Source: CAD feature listing. Evaluate the final solid. Frame: model axes, mm. Face numbers are marked on the shaded views. Coordinates: 2 decimals unless noted, no trailing zeros. Order: outer loops, then holes, each group sorted by start corner. A loop starts at its lowest first (then second) coordinate and runs counter-clockwise, first axis right, second up. Notation, with made-up numbers: (-1.5, 85.5) -> (5.5, 85.5) arc R30 cw to (5.5, 112.5) -> close; hole circle Ø8 at (25, -36). An arc over 180 degrees is marked (long way). Put each result on its own line as item: value.
from build123d import *

# Parameters (mm, degrees)
SKETCH1_R               = 12.5
SKETCH1_R_2             = 9.5
BOSS_EXTRUDE1_DEPTH     = 2
SKETCH1_3_R             = 9.5
SKETCH1_3_R_2           = 5
BOSS_EXTRUDE2_DEPTH     = 41.5
CUT_EXTRUDE1_REACH      = 47.108
CUT_EXTRUDE1_END_RADIUS = 9.5
SKETCH2_R               = 2.5


with BuildPart() as part:
    # Sketch1 → Boss-Extrude1 (new body)
    with BuildSketch(Plane.XY):
        Circle(SKETCH1_R)
        Circle(SKETCH1_R_2, mode=Mode.SUBTRACT)
    extrude(amount=BOSS_EXTRUDE1_DEPTH)

    # Sketch1<3> → Boss-Extrude2 (add)
    with BuildSketch(Plane.XY):
        Circle(SKETCH1_3_R)
        Circle(SKETCH1_3_R_2, mode=Mode.SUBTRACT)
    extrude(amount=BOSS_EXTRUDE2_DEPTH)

    # Cut-Extrude1: up to this cylinder (the profile starts inside it)
    cut_extrude1_end = Plane(origin=(0, 0, 17.5), z_dir=(0, 0, -1)) * Cylinder(CUT_EXTRUDE1_END_RADIUS, 114.216, mode=Mode.PRIVATE)
    # Sketch2 → Cut-Extrude1 (cut, up to the surface)
    with BuildSketch(Plane(origin=(0, 0, 0), x_dir=(1, 0, 0), z_dir=(0, 1, 0)), mode=Mode.PRIVATE) as cut_extrude1_sk1:
        with Locations(Location((0, -17.5, 0), (0, 0, 90))):
            Circle(SKETCH2_R)
    cut_extrude1_tool1 = extrude(cut_extrude1_sk1.sketch, amount=CUT_EXTRUDE1_REACH, mode=Mode.PRIVATE) & cut_extrude1_end
    add(cut_extrude1_tool1.solids().sort_by_distance((0, 0, 17.5))[0], mode=Mode.SUBTRACT)


solid = part.part
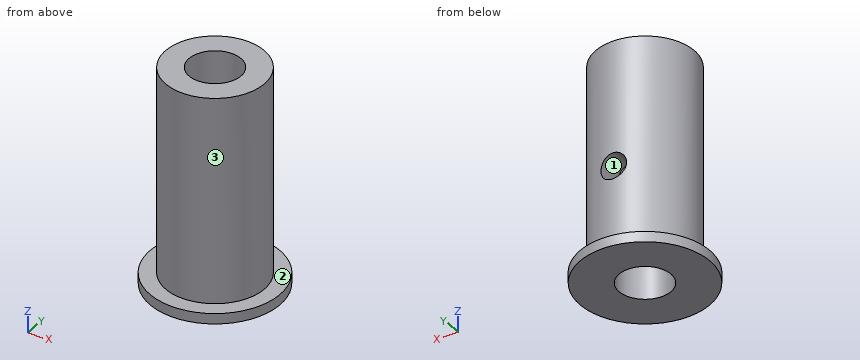
1. Cut plane B-B on x = -2. Output: boundary loops of the cut face in (y, z).
Numbers:
outline: (-12.34, 0) -> (-4.58, 0) -> (-4.58, 41.5) -> (-9.29, 41.5) -> (-9.29, 2) -> (-12.34, 2) -> close; (4.58, 0) -> (12.34, 0) -> (12.34, 2) -> (9.29, 2) -> (9.29, 16) -> (4.58, 16) -> close; (4.58, 19) -> (9.29, 19) -> (9.29, 41.5) -> (4.58, 41.5) -> close
2. Pull-direction query (Z, two-part tool) for the marked faces 1, 2 and 3; classes: pulls with the +Z half, pulls with the -Z half, needs draft (parallel to the pull), parting line crosses it, or undercut.
Numbers:
face 1: undercut
face 2: pulls with the +Z half
face 3: needs draft
3. Cut plane C-C on z = 29. Output: boundary loops of the cut face in (x, y).
Numbers:
outline: circle Ø19 at (0, 0); hole circle Ø10 at (0, 0)
4. Cut plane A-A on y = 8. Output: boundary loops of the cut face in (x, z), plus the area to 3 significant figures.
Numbers:
outline: (-9.6, 0) -> (9.6, 0) -> (9.6, 2) -> (5.12, 2) -> (5.12, 41.5) -> (-5.12, 41.5) -> (-5.12, 2) -> (-9.6, 2) -> close; hole circle Ø5 at (0, 17.5)
area: 424 mm2
5. Cut plane D-D on x = -6.5. Output: boundary loops of the cut face in (y, z).
Numbers:
outline: (-10.68, 0) -> (10.68, 0) -> (10.68, 2) -> (6.93, 2) -> (6.93, 41.5) -> (-6.93, 41.5) -> (-6.93, 2) -> (-10.68, 2) -> close
6. Ray query, line 1 along Y through (x, z) = (0, 13); line 2 along X through (y, z) = (8.4, 17.5); line 3 along Z through (x, y) = (-3.25, 10). Return the intervals inside material, ascending.
Numbers:
line 1: y = -9.5 to -5, 5 to 9.5
line 2: x = -4.44 to -2.5, 2.5 to 4.44
line 3: z = 0 to 2
7. First-contact query: pin 1 (3 mm diameter, centred on y = 6, z = 26, fed in from +X); pin 2 (8 mm diameter, centred on y = -7.5, z = 5.5, fed in from +X); pin 3 (6 mm diameter, centred on y = 4, z = 12, fed in from -X). Flat tips, straight axial feed; report the tip coordinate or a pass-through.
Numbers:
pin 1: stops at x = 8.37
pin 2: stops at x = 11.19
pin 3: stops at x = -9.45
